Geometry: final body of the model. Coordinates: model frame, mm. A direction names the side the tool comes from. Give positions to 0.01 mm unless a question says otherwise; leave off trailing zeros. Write each loop counter-clockwise with the first axis right and the second up, starting at its lowest first coordinate (ties: lowest second). Pieces come first, ordered by that corner, then holes.
from build123d import *

# Parameters (mm, degrees)
SKETCH_1_W           = 20
SKETCH_1_H           = 20
EXTRUDE_1_DEPTH      = 4
SKETCH_2_W           = 14
SKETCH_2_H           = 14
CUT_EXTRUDE_1_DEPTH  = 2
EXTRUDE_2_DEPTH      = 20
EXTRUDE_3_DEPTH      = 20
EXTRUDE_4_DEPTH      = 20
EXTRUDE_4_DEPTH_BACK = 4
SKETCH_7_R           = 1.8
CUT_EXTRUDE_5_DEPTH  = 41
SKETCH_8_R           = 1.8
CUT_EXTRUDE_6_DEPTH  = 20
SKETCH_9_R           = 1.8
CUT_EXTRUDE_7_DEPTH  = 20


with BuildPart() as part:
    # 草图1 → 凸台-拉伸1 (new body)
    with BuildSketch(Plane.XY):
        Rectangle(SKETCH_1_W, SKETCH_1_H)
    extrude(amount=EXTRUDE_1_DEPTH)

    # 草图2 → 切除-拉伸1 (cut)
    with BuildSketch(Plane(origin=(0, 0, 0), x_dir=(-1, 0, 0), z_dir=(0, 0, -1))):
        Rectangle(SKETCH_2_W, SKETCH_2_H)
    extrude(amount=-CUT_EXTRUDE_1_DEPTH, mode=Mode.SUBTRACT)

    # 草图3 → 凸台-拉伸2 (add)
    with BuildSketch(Plane(origin=(10, 0, 0), x_dir=(0, 0, -1), z_dir=(1, 0, 0))):
        Polygon((-4, -2), (-4, 2), (-2.5, 2), (-2.5, 3.9), (-0.9, 3.9), (0, 3), (0, -3), (-0.9, -3.9), (-2.5, -3.9), (-2.5, -2), align=None)
    extrude(amount=EXTRUDE_2_DEPTH)

    # 草图5 → 凸台-拉伸3 (add)
    with BuildSketch(Plane(origin=(0, 10, 0), x_dir=(1, 0, 0), z_dir=(0, 1, 0))):
        Polygon((2, -4), (-2, -4), (-2, -2.5), (-3.9, -2.5), (-3.9, -0.9), (-3, 0), (3, 0), (3.9, -0.9), (3.9, -2.5), (2, -2.5), align=None)
    extrude(amount=EXTRUDE_3_DEPTH)

    # 草图6 → 凸台-拉伸4 (add, two sides)
    with BuildSketch(Plane(origin=(0, 0, 0), x_dir=(-1, 0, 0), z_dir=(0, 0, -1))) as extrude_4_sk:
        Polygon((10, 2), (10, -2), (8.5, -2), (8.5, -3.9), (6.723155125, -3.9), (6, -3), (6, 3), (6.723155125, 3.9), (8.5, 3.9), (8.5, 2), align=None)
        Polygon((2, -10), (-2, -10), (-2, -8.5), (-3.9, -8.5), (-3.9, -6.853318906), (-3, -6), (3, -6), (3.9, -6.853318906), (3.9, -8.5), (2, -8.5), align=None)
    extrude(amount=EXTRUDE_4_DEPTH)
    extrude(extrude_4_sk.sketch, amount=-EXTRUDE_4_DEPTH_BACK)

    # 草图7 → 切除-拉伸5 (cut, through all)
    with BuildSketch(Plane.ZY.offset(10)):
        with Locations((-6, 0)):
            Circle(SKETCH_7_R)
        with Locations((-13, 0)):
            Circle(SKETCH_7_R)
    extrude(amount=-CUT_EXTRUDE_5_DEPTH, mode=Mode.SUBTRACT)

    # 草图8 → 切除-拉伸6 (cut)
    with BuildSketch(Plane(origin=(0, 0, 0), x_dir=(-1, 0, 0), z_dir=(0, 0, -1))):
        with Locations((-16, 0)):
            Circle(SKETCH_8_R)
        with Locations((0, 16)):
            Circle(SKETCH_8_R)
        with Locations((0, 23)):
            Circle(SKETCH_8_R)
        with Locations((-23, 0)):
            Circle(SKETCH_8_R)
    extrude(amount=-CUT_EXTRUDE_6_DEPTH, mode=Mode.SUBTRACT)

    # 草图9 → 切除-拉伸7 (cut)
    with BuildSketch(Plane.XZ.offset(10)):
        with Locations((0, -6)):
            Circle(SKETCH_9_R)
        with Locations((0, -13)):
            Circle(SKETCH_9_R)
    extrude(amount=-CUT_EXTRUDE_7_DEPTH, mode=Mode.SUBTRACT)


solid = part.part
Q1. Ray query, line 1 along Z through (x, y) = (0, -7.25); line 2 along Y through (x, z) = (16, 1.95); line 3 along X through (y, z) = (-5, 3). Return the intervals inside material, ascending.
Filled sheet:
line 1: z = -20 to -14.8, -11.2 to -7.8, -4.2 to 4
line 2: y = -3.9 to -1.8, 1.8 to 3.9
line 3: x = -10 to 10
Q2. Section A-A on y = 0. Output: boundary loops of the cut face in (x, z).
Filled sheet:
outline: (-10, -20) - (-6, -20) - (-6, -14.8) - (-10, -14.8) - close; (-10, -11.2) - (-6, -11.2) - (-6, -7.8) - (-10, -7.8) - close; (-10, -4.2) - (-6, -4.2) - (-6, 2) - (7, 2) - (7, 0) - (14.2, 0) - (14.2, 4) - (-10, 4) - close; (17.8, 0) - (21.2, 0) - (21.2, 4) - (17.8, 4) - close; (24.8, 0) - (30, 0) - (30, 4) - (24.8, 4) - close
Q3. Section D-D on z = -6. Output: boundary loops of the cut face in (x, y).
Filled sheet:
outline: (-10, -2) - (-8.5, -2) - (-8.5, -3.9) - (-6.72, -3.9) - (-6, -3) - (-6, -1.8) - (-10, -1.8) - close; (-10, 1.8) - (-6, 1.8) - (-6, 3) - (-6.72, 3.9) - (-8.5, 3.9) - (-8.5, 2) - (-10, 2) - close; (-3.9, -8.5) - (-2, -8.5) - (-2, -10) - (-1.8, -10) - (-1.8, -6) - (-3, -6) - (-3.9, -6.85) - close; (1.8, -10) - (2, -10) - (2, -8.5) - (3.9, -8.5) - (3.9, -6.85) - (3, -6) - (1.8, -6) - close
Q4. Access query for faces 1 (the flat face through (0, -6, -9)), 2 (the flat face through (30, 0, 2)), 3 (the flat face through (-8.5, -3, -10)), 4 (the flat face through (-3, 20, 2.5)), 5 (the flat face through (20, -3.9, 2)). Directions: +Z, -Z, +X, -X, +Y, -Y. A direction counts if a zero-diameter tool reaches every point of the face in a straight line with its end or side. Return the directions, or none.
Filled sheet:
face 1: -Z
face 2: +Z, -Z, +X, +Y, -Y
face 3: -Z, -X, -Y
face 4: +Z, -X, +Y
face 5: +Z, -Z, +X, -Y
Q5. Pin query (flat end, axial travel): P1, Ø6, axis at y = 25.5, z = 1, coming from the +X side; P2, Ø1.2, axis at y = -9.5, z = -11, coming from the +X side; P3, Ø0.6, axis at x = 21.5, y = -3.5, coming from the +Z side; P4, Ø2, axis at y = 0, z = -6, coming from the -X side. Return the tip coordinate at first contact, or that it passes through.
Filled sheet:
P1: stops at x = 3.9
P2: stops at x = 2
P3: stops at z = 2.5
P4: passes through
Q6. Pull-direction query (Y, two-part tool) for faces 6 (the flat face through (-5, -7, 1)), 7 (the cylindrical face through (0.234, 17.785, 1.972)), 8 (the flat face through (10, -7, 2)), 9 (the flat face through (20, 2, 3)); classes: released by +Y, released by -Y, zero draft, split by the parting line, or undercut.
Filled sheet:
face 6: undercut
face 7: undercut
face 8: zero draft
face 9: released by +Y
Q7. Section C-C on z = -9. Output: boundary loops of the cut face in (x, y).
Filled sheet:
outline: (-10, -2) - (-8.5, -2) - (-8.5, -3.9) - (-6.72, -3.9) - (-6, -3) - (-6, 3) - (-6.72, 3.9) - (-8.5, 3.9) - (-8.5, 2) - (-10, 2) - close; (-3.9, -8.5) - (-2, -8.5) - (-2, -10) - (2, -10) - (2, -8.5) - (3.9, -8.5) - (3.9, -6.85) - (3, -6) - (-3, -6) - (-3.9, -6.85) - close
